Verification items for the finished model (mm, model axes). A direction names the side the tool comes from. Give positions to 0.01 mm unless a question says otherwise; leave off trailing zeros. Write each loop counter-clockwise with the first axis right and the second up, starting at its lowest first coordinate (ties: lowest second). Pieces come first, ordered by that corner, then holes. Notation, with made-up numbers: (2, 11.25) - (21, 11.25) arc R19 ccw to (21, 27.25) - close; hole circle Ø7 at (-24.5, -5.75). An arc over 180 degrees is marked (long way). Answer as a JSON object with one key per item and string values. Group by question number.
Item 1: Tool access check on faces 1 (the face through (40, -8, 2)), 2 (the face through (0, -26.964, 2)). Record the directions out of +Z, -Z, +X, -X, +Y, -Y that give a thin tool (end or side, any length) a straight path to the whole face; none if there is none.
Item 2: Sectioned sample at C-C, the plane z = 1.3. Record the boundary of the cut face in (x, y) (3 decimals), and give its area (3 significant figures).
Item 3: Scan lines: line 1 along Y through (x, z) = (-31.5, 1.05) (3 decimals); line 2 along X through (y, z) = (-29, 2.5). Record each from-to range of solid material in increasing order. Write a range as [from, to].
Item 4: Draft check along X on faces 3 (the face through (-31, -31.814, 2)), 4 (the face through (31, -2.425, 2)), 5 (the face through (-40, -7, 2)), 6 (the face through (-1, 25, 2)). Enter one of: +X half, -X half, draft (parallel to the pull), parting line (faces both ways), or undercut.
Item 5: Sectioned sample at A-A, the plane x = -2.5. Record the boundary of the cut face in (y, z) (3 decimals).
Item 6: Sectioned sample at B-B, the plane y = -28. Record the boundary of the cut face in (x, z), and give its area (3 significant figures).
```python
from build123d import *

# Parameters (mm, degrees)
F0_W     = 80
F0_H     = 15
F0_W_2   = 10
F0_H_2   = 4.85
F0_W_3   = 20
F0_H_3   = 50
F1_DEPTH = 5


with BuildPart() as f1:
    # F0 (on Top) → F1 (new body)
    with BuildSketch(Plane.XY):
        with Locations((0, -32.5)):
            Rectangle(F0_W, F0_H)
        with Locations((-31, -29.389005)):
            Rectangle(F0_W_2, F0_H_2, mode=Mode.SUBTRACT)
        with Locations((0, -29.389005)):
            Rectangle(F0_W_3, F0_H_2, mode=Mode.SUBTRACT)
        with Locations((31, -29.389005)):
            Rectangle(F0_W_2, F0_H_2, mode=Mode.SUBTRACT)
        Rectangle(F0_W, F0_H_3)
        with Locations((-31, 0)):
            Rectangle(F0_W_2, F0_H_2, mode=Mode.SUBTRACT)
        Rectangle(F0_W_3, F0_H_2, mode=Mode.SUBTRACT)
        with Locations((31, 0)):
            Rectangle(F0_W_2, F0_H_2, mode=Mode.SUBTRACT)
    extrude(amount=F1_DEPTH)


solid = f1.part
```
Geometry check:
{
 "1": {"face 1": "+Z, -Z, +X, +Y, -Y", "face 2": "+Z, -Z"},
 "2": {"outline": "(-40, -40) - (40, -40) - (40, 25) - (-40, 25) - close; hole (-36, -31.814) - (-26, -31.814) - (-26, -26.964) - (-36, -26.964) - close; hole (-36, -2.425) - (-26, -2.425) - (-26, 2.425) - (-36, 2.425) - close; hole (-10, -31.814) - (10, -31.814) - (10, -26.964) - (-10, -26.964) - close; hole (-10, -2.425) - (10, -2.425) - (10, 2.425) - (-10, 2.425) - close; hole (26, -31.814) - (36, -31.814) - (36, -26.964) - (26, -26.964) - close; hole (26, -2.425) - (36, -2.425) - (36, 2.425) - (26, 2.425) - close", "area": "4,810 mm^2"},
 "3": {"line 1": "[-40, -31.814], [-26.964, -2.425], [2.425, 25]", "line 2": "[-40, -36], [-26, -10], [10, 26], [36, 40]"},
 "4": {"face 3": "undercut", "face 4": "undercut", "face 5": "-X half", "face 6": "draft"},
 "5": {"outline": "(-40, 0) - (-31.814, 0) - (-31.814, 5) - (-40, 5) - close; (-26.964, 0) - (-2.425, 0) - (-2.425, 5) - (-26.964, 5) - close; (2.425, 0) - (25, 0) - (25, 5) - (2.425, 5) - close"},
 "6": {"outline": "(-40, 0) - (-36, 0) - (-36, 5) - (-40, 5) - close; (-26, 0) - (-10, 0) - (-10, 5) - (-26, 5) - close; (10, 0) - (26, 0) - (26, 5) - (10, 5) - close; (36, 0) - (40, 0) - (40, 5) - (36, 5) - close", "area": "200 mm^2"}
}
